Work out the finished part from the listing and answer in its coordinate system (mm). A direction names the side the tool comes from. Give positions to 0.01 mm unless a question says otherwise; leave off trailing zeros. Loops run counter-clockwise (first coordinate to the right, second up) from the corner with the lowest first, then second, coordinate; pieces in that order, holes last. Notation, with made-up numbers: (-21, 0) - (36, 0) arc R24 cw to (36, 23) - close; hole circle Ø3 at (-20.5, -34). An arc over 180 degrees is marked (long way). One line per item, written item: value.
from build123d import *

# Parameters (mm, degrees)
F2_W     = 113.5670877993
F2_H     = 81.1927579343
F2_R     = 31.9732071905
F2_W_2   = 53.6017529666
F2_H_2   = 28.8779456168
F3_DEPTH = 25
F5_DEPTH = 25
F7_DEPTH = 7


with BuildPart() as f1:
    # F0 (on Front) → F1 (revolve)
    with BuildSketch(Plane.XZ):
        Polygon((-5.95, -0.4022617794), (-31.9732071905, -0.4022617794), (-31.9732071905, -7.4022617794), (-4, -7.4022617794), (-4, -5.9022617794), (-5.95, -5.9022617794), align=None)
    revolve(axis=Axis((0, 0, -6.3669939991), (0, 0, 1)))

    # F2 (on face) → F3 (cut)
    with BuildSketch(Plane(origin=(0, 0, -7.4022617794), x_dir=(1, 0, 0), z_dir=(0, 0, -1))):
        with Locations((1.571347937, -4.5206267387)):
            Rectangle(F2_W, F2_H)
        Circle(F2_R, mode=Mode.SUBTRACT)
        Circle(F2_R)
        Rectangle(F2_W_2, F2_H_2, mode=Mode.SUBTRACT)
    extrude(amount=-F3_DEPTH, mode=Mode.SUBTRACT)

    # F4 (on face) → F5 (cut)
    with BuildSketch(Plane(origin=(0, 0, -7.4022617794), x_dir=(1, 0, 0), z_dir=(0, 0, -1))):
        with BuildLine():
            Line((-3.9686269666, 0.5), (-9.2835435644, 0.5))
            Line((-9.2835435644, 0.5), (-9.2835435644, 6))
            Line((-9.2835435644, 6), (-26.8008764833, 6))
            Line((-26.8008764833, 6), (-26.8008764833, -6))
            Line((-26.8008764833, -6), (-9.2835435644, -6))
            Line((-9.2835435644, -6), (-9.2835435644, -0.5))
            Line((-9.2835435644, -0.5), (-3.9686269666, -0.5))
            ThreePointArc((-3.9686269666, -0.5), (-4, 0), (-3.9686269666, 0.5))
        make_face()
        with BuildLine():
            Line((9.2835435644, 0.5), (3.9686269666, 0.5))
            ThreePointArc((3.9686269666, 0.5), (3.9921490369, 0.2504916502), (4, 0))
            ThreePointArc((4, 0), (3.9921490369, -0.2504916502), (3.9686269666, -0.5))
            Line((3.9686269666, -0.5), (9.2835435644, -0.5))
            Line((9.2835435644, -0.5), (9.2835435644, -6))
            Line((9.2835435644, -6), (26.8008764833, -6))
            Line((26.8008764833, -6), (26.8008764833, 6))
            Line((26.8008764833, 6), (9.2835435644, 6))
            Line((9.2835435644, 6), (9.2835435644, 0.5))
        make_face()
    extrude(amount=-F5_DEPTH, mode=Mode.SUBTRACT)

    # F6 (on face) → F7 (join, through all)
    with BuildSketch(Plane(origin=(0, 0, -7.4022617794), x_dir=(1, 0, 0), z_dir=(0, 0, -1))):
        with BuildLine():
            Line((-21.8008764833, 6), (-23.8008764833, 6))
            add(Edge.make_bspline(
                [(-23.8008764833, 6), (-22.2108428095, 4.7094736127), (-19.3347207095, 3.1365293538), (-23.8174722022, -0.0420631575), (-28.2006493816, -2.9682767239), (-25.523675908, -5.0459788725), (-23.8008764833, -6)],
                knots=[0, 0, 0, 0, 0.25, 0.5, 0.75, 1, 1, 1, 1], degree=3))
            Line((-23.8008764833, -6), (-21.8008764833, -6))
            add(Edge.make_bspline(
                [(-21.8008764833, 6), (-20.2684628372, 5.0384721173), (-17.3238246823, 2.9890179574), (-21.7691782562, -0.0192710268), (-26.4047211931, -2.9119338502), (-23.0797043121, -5.1926403316), (-21.8008764833, -6)],
                knots=[0, 0, 0, 0, 0.25, 0.5, 0.75, 1, 1, 1, 1], degree=3))
        make_face()
        with BuildLine():
            add(Edge.make_bspline(
                [(23.8008764833, 6), (22.2108428095, 4.7094736127), (19.3347207095, 3.1365293538), (23.8174722022, -0.0420631575), (28.2006493816, -2.9682767239), (25.523675908, -5.0459788725), (23.8008764833, -6)],
                knots=[0, 0, 0, 0, 0.25, 0.5, 0.75, 1, 1, 1, 1], degree=3))
            Line((23.8008764833, 6), (21.8008764833, 6))
            add(Edge.make_bspline(
                [(21.8008764833, 6), (20.2684628372, 5.0384721173), (17.3238246823, 2.9890179574), (21.7691782562, -0.0192710268), (26.4047211931, -2.9119338502), (23.0797043121, -5.1926403316), (21.8008764833, -6)],
                knots=[0, 0, 0, 0, 0.25, 0.5, 0.75, 1, 1, 1, 1], degree=3))
            Line((21.8008764833, -6), (23.8008764833, -6))
        make_face()
    extrude(amount=-F7_DEPTH)


solid = f1.part
1. Find the intervals of material crossed by line 1 along Y through (x, z) = (15, -4.5); line 2 along Y through (x, z) = (-4, -6.75); line 3 along Y through (x, z) = (-23.5, -1.25), in increasing order.
Output:
line 1: y = -14.44 to -6, 6 to 14.44
line 2: y = -14.44 to -0.5, 0.5 to 14.44
line 3: y = -14.44 to -5.76, -0.21 to 1.16, 4.81 to 14.44
2. Section A-A (x = -8) is taken. Write down the section's boundary in (y, z).
Output:
outline: (-14.44, -7.4) - (-0.5, -7.4) - (-0.5, -0.4) - (-14.44, -0.4) - close; (0.5, -7.4) - (14.44, -7.4) - (14.44, -0.4) - (0.5, -0.4) - close
3. Flat-ended cylindrical pins translate along their axes: pin 1 Ø3 at (y, z) = (-3, -2.5) entering from -X; pin 2 Ø1 at (y, z) = (4.5, -6) entering from +X; pin 3 Ø1 at (y, z) = (-11.5, -3.5) entering from -X; pin 4 Ø12 at (x, y) = (9.5, -2) entering from +Z. Find the tip coordinate at first contact, or state that the pin passes through.
Output:
pin 1: stops at x = -21.86
pin 2: stops at x = 26.44
pin 3: stops at x = -26.8
pin 4: stops at z = -0.4
4. Section B-B (x = 17.5) is taken. Write down the section's boundary in (y, z), and give its area (3 significant figures).
Output:
outline: (-14.44, -7.4) - (-6, -7.4) - (-6, -0.4) - (-14.44, -0.4) - close; (6, -7.4) - (14.44, -7.4) - (14.44, -0.4) - (6, -0.4) - close
area: 118 mm²
5. For faces 4 (the flat face through (-0.1, 4.4, -5.902)), 5 (the flat face through (26.801, -10, -4)), 6 (the flat face through (7, -3, -7.402)), 7 (the cylindrical face through (0, 4, -7)), 8 (the flat face through (-25, -6, -4)), determine the directions among +Z, -Z, +X, -X, +Y, -Y from which every point of the face is accessible in a straight line to the end or side of a thin tool.
Output:
face 4: +Z
face 5: +Z, -Z, +X, +Y, -Y
face 6: -Z, +X, -X, +Y, -Y
face 7: +Z, -Z
face 8: +Z, -Z, -X
6. Section C-C (y = 5) is taken. Count the separate pieces of the cut face and the enclosed holes in it, and give its area (3 significant figures).
Output:
separate pieces: 3
enclosed holes: 0
area: 124 mm²
7. The mould has two halves that part along Y. Classify faces 1 (the flat face through (25, 6, -4)), 2 (the flat face through (-26.801, -10, -4)), 3 (the flat face through (0, -14.439, -4)): released by +Y, released by -Y, zero draft, split by the parting line, or undercut.
Output:
face 1: undercut
face 2: zero draft
face 3: released by -Y
